from build123d import *
from build123d import SkipClean  # not in build123d's __all__

# Parameters (mm, degrees)
F0_W     = 100
F0_H     = 15
F1_DEPTH = 40
F0_R     = 18
F2_DEPTH = 5
F3_DEPTH = 30
F5_DEPTH = 5


# Not quite as in the source:
# - a pattern or mirror of a feature is missing from the dataset's text; its kind, count and spacing are read off the source's solid


with BuildPart() as f1:
    # F0 (on Front) → F1 (new body, symmetric)
    with BuildSketch(Plane.XZ):
        with Locations((0, 7.5)):
            Rectangle(F0_W, F0_H)
    extrude(amount=F1_DEPTH, both=True)

    # F0 (on Front) → F2 (join, symmetric)
    with BuildSketch(Plane.XZ):
        with BuildLine():
            ThreePointArc((-30, 75), (-35.1316701949, 43.3772233983), (-50, 15))
            Line((-50, 15), (50, 15))
            ThreePointArc((50, 15), (35.1316701949, 43.3772233983), (30, 75))
            ThreePointArc((30, 75), (0, 45), (-30, 75))
        make_face()
        with Locations((0, 7.5)):
            Rectangle(F0_W, F0_H)
        with BuildLine():
            ThreePointArc((30, 75), (0, 105), (-30, 75))
            ThreePointArc((-30, 75), (0, 45), (30, 75))
        make_face()
        with Locations((0, 75)):
            Circle(F0_R, mode=Mode.SUBTRACT)
    extrude(amount=F2_DEPTH, both=True)

    # F0 (on Front) → F3 (join, symmetric)
    with BuildSketch(Plane.XZ):
        with BuildLine():
            ThreePointArc((30, 75), (0, 105), (-30, 75))
            ThreePointArc((-30, 75), (0, 45), (30, 75))
        make_face()
        with Locations((0, 75)):
            Circle(F0_R, mode=Mode.SUBTRACT)
    with SkipClean():  # cleaning this boolean's faces spoils the solid; the shape is the same uncleaned
        extrude(amount=F3_DEPTH, both=True)

    # F4 (on Right) → F5 (join, symmetric)
    with BuildSketch(Plane.YZ):
        with BuildLine():
            ThreePointArc((40, 15), (33.4008913624, 29.4669637875), (30, 45))
            Line((30, 45), (30, 50))
            Line((30, 50), (5, 50))
            Line((5, 50), (5, 15))
            Line((5, 15), (40, 15))
        make_face()
    f5 = extrude(amount=F5_DEPTH, both=True)

    # F5_copies: F5 across plane
    add(f5.mirror(Plane(origin=(0, 0, 0), x_dir=(0, 0, -1), z_dir=(0, -1, 0))), clean=False)


solid = f1.part
CAD build for the part. Positions are in the model's coordinates, mm. A direction names the side the tool comes from. Round coordinates to 2 decimals unless told otherwise and drop trailing zeros. Order: outer loops, then holes, each group sorted by start corner. A loop starts at its lowest first (then second) coordinate and runs counter-clockwise, first axis right, second up. Notation, with made-up numbers: (12.25, -39) -> (63.25, -39) arc R15 cw to (63.25, -35) -> close; hole circle Ø11 at (60.25, -8.75). An arc over 180 degrees is marked (long way). Write each question's results on one line, items separated by ' | '.
1. Flat gauge pins, fed straight in: P1, Ø17.5, axis at x = 19.5, y = -14, coming from the +Z side; P2, Ø12, axis at x = -20.5, z = 78.5, coming from the -Y side; P3, Ø9, axis at y = 20, z = 33, coming from the -X side. Where does each tip first touch, or does it go through?
Findings below:
P1: stops at z = 103.01 | P2: stops at y = -30 | P3: stops at x = -5
2. Cut at D-D (z = 19). Give the cut face in (x, y).
Findings below:
outline: (-47.15, -5) -> (-5, -5) -> (-5, -37.8) -> (5, -37.8) -> (5, -5) -> (47.15, -5) -> (47.15, 5) -> (5, 5) -> (5, 37.8) -> (-5, 37.8) -> (-5, 5) -> (-47.15, 5) -> close
3. Wall check: line 1 along Z through (x, y) = (0, 2); line 2 along Y through (x, z) = (-24, 36); line 3 along Y through (x, z) = (22.5, 76.5). Give the ranges that are in metal, low to high. Write a range as [from, to].
Findings below:
line 1: z = [0, 57], [93, 105] | line 2: y = [-5, 5] | line 3: y = [-30, 30]
4. 3-axis set-ups, long thin cutter, end or side, ignore diameter. For faces 4 (the face through (5, -18, 30)), 5 (the face through (27, 22, 15)), 6 (the face through (-13, 30, 88)), 7 (the face through (-28, 22, 15)): which of +Z, -Z, +X, -X, +Y, -Y reach the whole face in a straight line?
Findings below:
face 4: +X, -Y | face 5: +X, +Y | face 6: +Z, +X, -X, +Y | face 7: -X, +Y
5. Cut at C-C (x = -22.5). Give the cut face in (y, z), plus the area to 3 significant figures.
Findings below:
outline: (-40, 0) -> (40, 0) -> (40, 15) -> (5, 15) -> (5, 55.16) -> (30, 55.16) -> (30, 94.84) -> (-30, 94.84) -> (-30, 55.16) -> (-5, 55.16) -> (-5, 15) -> (-40, 15) -> close | area: 3,980 mm²
6. Pull direction Z, two halves, no side cores. Call faces 1 (the face through (-13, -30, 88)), 2 (the face through (-5, 18, 30)), 3 (the face through (0.07, -33.47, 29.26)): pulls with the +Z half, pulls with the -Z half, needs draft (parallel to the pull), parting line crosses it, or undercut.
Findings below:
face 1: needs draft | face 2: undercut | face 3: pulls with the +Z half
7. Cut at B-B (y = -14.5). Give the cut face in (x, z), plus the area to 3 significant figures.
Findings below:
outline: (-50, 0) -> (50, 0) -> (50, 15) -> (5, 15) -> (5, 45.42) arc R30 ccw (long way) to (-5, 45.42) -> (-5, 15) -> (-50, 15) -> close; hole circle Ø36 at (0, 75) | area: 3,610 mm²
8. Cut at A-A (x = 0). Give the cut face in (y, z).
Findings below:
outline: (-40, 0) -> (40, 0) -> (40, 15) arc R75 cw to (30, 45) -> (30, 57) -> (-30, 57) -> (-30, 45) arc R75 cw to (-40, 15) -> close; (-30, 93) -> (30, 93) -> (30, 105) -> (-30, 105) -> close
